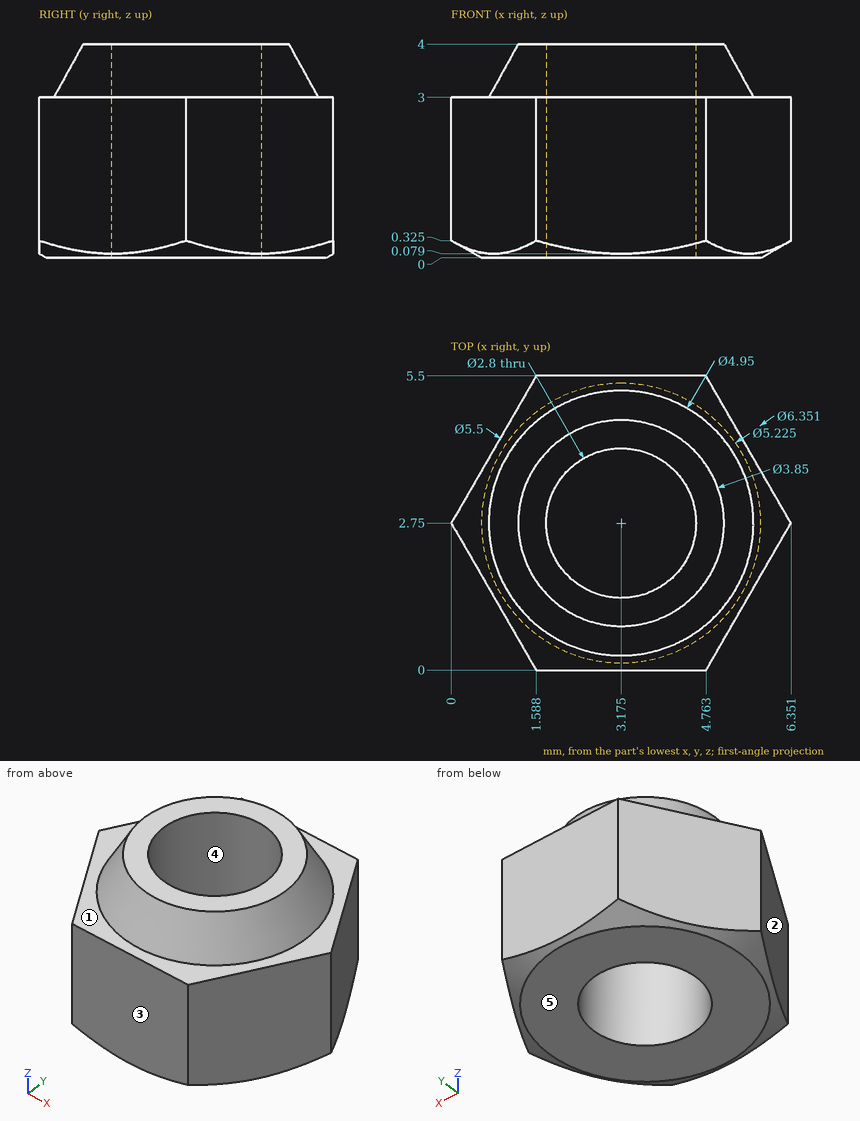
Part print with two shaded views. Sizes in mm from the minimum x, y, z corner. A direction names the side the tool comes from. Give positions to 0.01 mm unless a question says otherwise; leave off trailing zeros.
1) Wall check: probe 1 along Y at (x, z) = (3.25, 2.15); probe 2 along Z at (x, y) = (5.5, 1.75); probe 3 along X at (y, z) = (2.75, 3.1) (1 decimal). Give the ranges that are in metal, low to high.
2) Mould opens along Y. For the marked faces 3, 4 and 5 say: +Y half, -Y half, draft (parallel to the pull), parting line (faces both ways), or undercut.
3) 3-axis set-ups, long thin cutter, end or side, ignore diameter. For the marked faces 1 and 2: which of +Z, -Z, +X, -X, +Y, -Y reach the whole face in a straight line?
Computed:
1. probe 1: y = 0 to 1.35, 4.15 to 5.5
1. probe 2: z = 0 to 3
1. probe 3: x = 0.8 to 1.8, 4.6 to 5.6
2. face 3: -Y half
2. face 4: undercut
2. face 5: draft
3. face 1: +Z
3. face 2: +Z, -Z, -X, -Y
